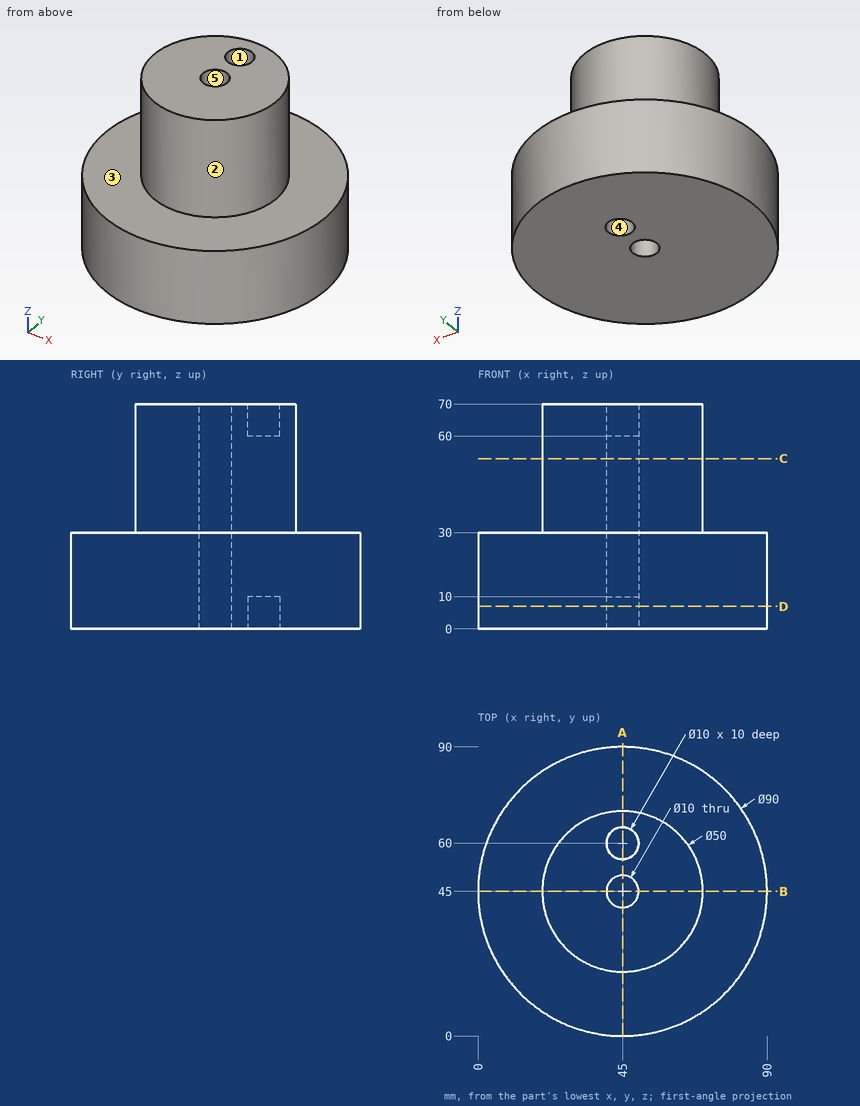
Can you work these out from the drawing? Everything is in mm from the part's minimum corner. A direction names the side the tool comes from. Coordinates: 2 decimals unless noted, no trailing zeros. Order: outer loops, then holes, each group sorted by start corner. A loop starts at its lowest first (then second) coordinate and runs counter-clockwise, first axis right, second up. Notation, with made-up numbers: (10.5, 2.25) -> (53.5, 2.25) arc R29 cw to (53.5, 29.25) -> close; hole circle Ø1 at (64.5, -28). An arc over 180 degrees is marked (long way). Use one line per item in the form item = value.
Q1. Which directions (+Z, -Z, +X, -X, +Y, -Y) give clear straight access to the entire face, cutting with the end or side of a thin tool? Please do the marked faces 4 and 5.
From the geometry:
face_4 = -Z
face_5 = +Z, -Z
Q2. Imagine slicing it at A-A, the plane x = 45. List the corners of the cut face in (y, z) for me.
From the geometry:
outline = (0, 0) -> (40, 0) -> (40, 70) -> (20, 70) -> (20, 30) -> (0, 30) -> close; (50, 0) -> (55, 0) -> (55, 10) -> (65, 10) -> (65, 0) -> (90, 0) -> (90, 30) -> (70, 30) -> (70, 70) -> (65, 70) -> (65, 60) -> (55, 60) -> (55, 70) -> (50, 70) -> close
Q3. Imagine slicing it at D-D, the plane z = 7. List the corners of the cut face in (x, y) for me.
From the geometry:
outline = circle Ø90 at (45, 45); hole circle Ø10 at (45, 45); hole circle Ø10 at (45, 60)
Q4. Imagine slicing it at B-B, the plane y = 45. List the corners of the cut face in (x, z) for me.
From the geometry:
outline = (0, 0) -> (40, 0) -> (40, 70) -> (20, 70) -> (20, 30) -> (0, 30) -> close; (50, 0) -> (90, 0) -> (90, 30) -> (70, 30) -> (70, 70) -> (50, 70) -> close
Q5. Imagine slicing it at C-C, the plane z = 53. List the corners of the cut face in (x, y) for me, then the cut area to 3 significant figures.
From the geometry:
outline = circle Ø50 at (45, 45); hole circle Ø10 at (45, 45)
area = 1,880 mm²
Q6. We'd pull the mould along Y, two halves only. Please class the marked faces 1, 2 and 3: released by +Y, released by -Y, zero draft, split by the parting line, or undercut.
From the geometry:
face_1 = undercut
face_2 = split by the parting line
face_3 = zero draft
Q7. I need wall thicknesses on L1, parallel to Y at x = 45, z = 3; L2, parallel to Y at x = 45, z = 17; L3, parallel to Z at x = 20, y = 57. Which ranges of each line are inside material? Lowest first, please.
From the geometry:
L1 = 0 to 40, 50 to 55, 65 to 90
L2 = 0 to 40, 50 to 90
L3 = 0 to 30
Q8. Will these pins go through, and if not, where does the flat tip stop? P1, Ø11.5, axis at x = 45, y = 60, coming from the -Z side; P2, Ø8, axis at x = 45, y = 60, coming from the -Z side; P3, Ø6, axis at y = 33.5, z = 49.5, coming from the +X side; P4, Ø1.5, axis at x = 58, z = 18, coming from the -Y side.
From the geometry:
P1 = 0
P2 = 10
P3 = 68.51
P4 = 1.7
